Work out the finished part from the listing and answer in its coordinate system (mm). Round coordinates to 2 decimals unless told otherwise and drop trailing zeros. Write each loop counter-clockwise with the first axis right and the second up, starting at its lowest first coordinate (ties: lowest second). Pieces come first, ordered by that corner, then holes. Notation, with made-up numbers: M -6.75,-24 L 11.25,-24 A26 ccw 11.25,-5 Z; hole C 65.25,53 d10. An arc over 180 degrees is marked long. Answer in a Markdown table with one row per item.
```python
from build123d import *

# Parameters (mm, degrees)
SKETCH1_R           = 17.78
BOSS_EXTRUDE1_DEPTH = 35.56
SKETCH2_R           = 10.5
CUT_EXTRUDE1_DEPTH  = 1
CHAMFER1_SIZE       = 0.635
CHAMFER2_SIZE       = 0.635


with BuildPart() as part:
    # Sketch1 → Boss-Extrude1 (new body)
    with BuildSketch(Plane.XZ):
        Circle(SKETCH1_R)
    extrude(amount=-BOSS_EXTRUDE1_DEPTH)

    # Sketch2 → Cut-Extrude1 (cut)
    with BuildSketch(Plane.XZ):
        Circle(SKETCH2_R)
    extrude(amount=-CUT_EXTRUDE1_DEPTH, mode=Mode.SUBTRACT)

    # Chamfer1
    chamfer1_edges = [part.edges().sort_by_distance(p)[0] for p in [
        (-17.78, 0, 0),
    ]]
    chamfer(chamfer1_edges, length=CHAMFER1_SIZE)

    # Chamfer2
    chamfer2_edges = [part.edges().sort_by_distance(p)[0] for p in [
        (-17.78, 35.56, 0),
    ]]
    chamfer(chamfer2_edges, length=CHAMFER2_SIZE)


solid = part.part
```
1. The part is cut by section C-C (y = 3). Determine the outline of the cut face in (x, z).
Calculated:
| item | result |
|---|---|
| outline | C 0,0 d35.56 |
2. Given pin 1 (6 mm diameter, centred on y = 22.5, z = -11, fed in from -X); pin 2 (5 mm diameter, centred on x = -4.5, y = 13, fed in from -Z); pin 3 (1 mm diameter, centred on x = 10.5, y = 17, fed in from -Z), each flat-ended and moving along its own axis, determine where each tip first touches the part or whether it passes through.
Calculated:
| item | result |
|---|---|
| pin 1 | stops at x = -15.88 |
| pin 2 | stops at z = -17.67 |
| pin 3 | stops at z = -14.7 |
3. Determine the mould class of faces 1 (the cylindrical face through (-3.85, 17.54, -17.36)), 2 (the flat face through (0, 1, 0)), 3 (the cylindrical face through (10, 0.5, 3.2)), 4 (the flat face through (7.4, 0, 7.9)) for opening direction Z: released by +Z, released by -Z, zero draft, split by the parting line, or undercut.
Calculated:
| item | result |
|---|---|
| face 1 | split by the parting line |
| face 2 | undercut |
| face 3 | undercut |
| face 4 | zero draft |
4. Consider line 1 along Z through (x, y) = (0, 0.75); line 2 along Y through (x, z) = (6, -6); line 3 along Z through (x, y) = (0, 0.6) (3 decimals). Determine where each line is inside the solid, lowest interval first. Write a range as from..to.
Calculated:
| item | result |
|---|---|
| line 1 | z = -17.78..-10.5, 10.5..17.78 |
| line 2 | y = 1..35.56 |
| line 3 | z = -17.745..-10.5, 10.5..17.745 |
5. The part is cut by section B-B (x = 0). Determine the outline of the cut face in (y, z) (3 decimals), plus the area to 3 significant figures.
Calculated:
| item | result |
|---|---|
| outline | M 0,-17.145 L 0.635,-17.78 L 34.925,-17.78 L 35.56,-17.145 L 35.56,17.145 L 34.925,17.78 L 0.635,17.78 L 0,17.145 L 0,10.5 L 1,10.5 L 1,-10.5 L 0,-10.5 Z |
| area | 1,240 mm² |
6. The part is cut by section A-A (z = 0). Determine the outline of the cut face in (x, y) (3 decimals).
Calculated:
| item | result |
|---|---|
| outline | M -17.78,0.635 L -17.145,0 L -10.5,0 L -10.5,1 L 10.5,1 L 10.5,0 L 17.145,0 L 17.78,0.635 L 17.78,34.925 L 17.145,35.56 L -17.145,35.56 L -17.78,34.925 Z |
